Input: part model. Units: mm. Frame: model coordinates. A direction names the side the tool comes from. Coordinates: 2 decimals unless noted, no trailing zeros. Loops run counter-clockwise (first coordinate to the right, second up) from the corner with the lowest first, then second, coordinate; pieces in that order, holes last. Notation, with made-up numbers: M -16,-13.5 L -12,-13.5 A26 cw -12,13.5 Z; hole C 23,39 d11. An arc over 180 degrees is marked long. Use a Markdown table: item, result. Add a question column.
1. Set-up query: faces 1 (the flat face through (0, 0, 11)), 2 (the flat face through (0, -0.75, 1)). Return all of +Z, -Z, +X, -X, +Y, -Y with unobstructed straight access to the full face (end or side cutting, diameter ignored); none if empty.
2. Draft query along Y for faces 3 (the flat face through (0, 0.75, 1)), 4 (the cylindrical face through (-0.27, -1.22, 6.56)), 5 (the flat face through (-2, 0, 2)), 6 (the flat face through (0, 0, 1.5)). Return one class per face: +Y half, -Y half, draft (parallel to the pull), parting line (faces both ways), or undercut.
3. Line query: L1, parallel to X at y = 0.5, z = 6.75; L2, parallel to X at y = 0.9, z = 9.25. Output: solid intervals per line, ascending. Write a range as [from, to].
4. Pin query (flat end, axial travel): pin 1 (1 mm diameter, centred on x = -2, y = 0.5, fed in from +Z); pin 2 (1 mm diameter, centred on x = 0, z = 5, fed in from +Y); pin 3 (2 mm diameter, centred on x = -1.5, z = 2.5, fed in from +Y). Return the tip coordinate at first contact, or that it passes through.
5. Section A-A on z = 2.5. Output: boundary loops of the cut face in (x, y), then the cut area to 3 significant figures.
```python
from build123d import *

# Parameters (mm, degrees)
F1_R     = 2.5
F1_R_2   = 1.25
F2_DEPTH = 2
F3_START = 1.5
F3_DEPTH = 0.5
F4_START = 2
F4_DEPTH = 9
F5_SIZE2 = 1.25
F5_SIZE  = 1.25
F6_R     = 0.25


# Not quite as in the source:
# - a feature names something its author has since deleted; it is built from what else it names


with BuildPart() as f2:
    # F1 (on Top) → F2 (new body)
    with BuildSketch(Plane.XY):
        Circle(F1_R)
        Circle(F1_R_2, mode=Mode.SUBTRACT)
        Circle(F1_R_2)
        Polygon((-0.4330127019, -0.75), (-0.8660254038, 0), (-0.4330127019, 0.75), (0.4330127019, 0.75), (0.8660254038, 0), (0.4330127019, -0.75), align=None, mode=Mode.SUBTRACT)
    extrude(amount=F2_DEPTH)

    # F1 (on Top) → F3 (join)
    with BuildSketch(Plane.XY.offset(F3_START)):
        Polygon((-0.4330127019, 0.75), (-0.8660254038, 0), (-0.4330127019, -0.75), (0.4330127019, -0.75), (0.8660254038, 0), (0.4330127019, 0.75), align=None)
    extrude(amount=F3_DEPTH)

    # F1 (on Top) → F4 (join)
    with BuildSketch(Plane.XY.offset(F4_START)):
        Circle(F1_R_2)
        Polygon((-0.4330127019, -0.75), (-0.8660254038, 0), (-0.4330127019, 0.75), (0.4330127019, 0.75), (0.8660254038, 0), (0.4330127019, -0.75), align=None, mode=Mode.SUBTRACT)
        Polygon((-0.4330127019, 0.75), (-0.8660254038, 0), (-0.4330127019, -0.75), (0.4330127019, -0.75), (0.8660254038, 0), (0.4330127019, 0.75), align=None)
    extrude(amount=F4_DEPTH)

    # F5
    f5_edges = [f2.edges().sort_by_distance(p)[0] for p in [
        (-2.5, 0, 0),
    ]]
    chamfer(f5_edges, length=F5_SIZE, length2=F5_SIZE2)

    # F6
    f6_edges = [f2.edges().sort_by_distance(p)[0] for p in [
        (-2.5, 0, 2),
        (-1.25, 0, 2),
        (-1.25, 0, 0),
        (-2.5, 0, 1.25),
    ]]
    fillet(f6_edges, radius=F6_R)


solid = f2.part
```
Answers below:
| question | item | result |
|---|---|---|
| 1 | face 1 | +Z, +X, -X, +Y, -Y |
| 1 | face 2 | -Z |
| 2 | face 3 | undercut |
| 2 | face 4 | parting line |
| 2 | face 5 | draft |
| 2 | face 6 | undercut |
| 3 | L1 | x = [-1.15, 1.15] |
| 3 | L2 | x = [-0.87, 0.87] |
| 4 | pin 1 | stops at z = 2 |
| 4 | pin 2 | stops at y = 1.25 |
| 4 | pin 3 | stops at y = 2.37 |
| 5 | outline | C 0,0 d2.5 |
| 5 | area | 4.91 mm² |
